Geometry: final body of the model. Coordinates: model frame, mm. Face numbers are marked on the shaded views. A direction names the side the tool comes from. Coordinates: 2 decimals unless noted, no trailing zeros. Loops run counter-clockwise (first coordinate to the right, second up) from the corner with the lowest first, then second, coordinate; pieces in that order, holes last. Notation, with made-up numbers: (57, -27.5) - (104, -27.5) arc R19 ccw to (104, -18.5) - close; hole circle Ø5 at (22.25, -1). An arc over 180 degrees is marked (long way). Answer in a Markdown table with one row per item.
from build123d import *

# Parameters (mm, degrees)
ESBO_O1_R                     = 7.7
ESBO_O1_R_2                   = 5.7
RESSALTO_EXTRUS_O1_DEPTH      = 40
RESSALTO_EXTRUS_O3_DEPTH      = 1
RESSALTO_EXTRUS_O3_DEPTH_BACK = 2
ESBO_O4_R                     = 1.65
CORTE_EXTRUS_O1_DEPTH         = 9.7
ESBO_O5_W                     = 3.890243015
ESBO_O5_H                     = 2
RESSALTO_EXTRUS_O4_DEPTH      = 40
PADR_OCIRCULAR1_COUNT         = 10
ESBO_O6_R                     = 5.3
CORTE_EXTRUS_O2_DEPTH         = 41


with BuildPart() as part:
    # Esboço1 → Ressalto-extrusão1 (new body)
    with BuildSketch(Plane.XY):
        Circle(ESBO_O1_R)
        Circle(ESBO_O1_R_2, mode=Mode.SUBTRACT)
    extrude(amount=RESSALTO_EXTRUS_O1_DEPTH)

    # Esboço3 → Ressalto-extrusão3 (add, two sides)
    with BuildSketch(Plane(origin=(0, 0, 0), x_dir=(1, 0, 0), z_dir=(0, 1, 0))) as ressalto_extrus_o3_sk:
        Polygon((7.7, -40), (13.7, -35), (13.7, -29), (7.7, -24), (6.7, -24), (6.7, -40), align=None)
        Polygon((7.7, 0), (13.7, -5), (13.7, -11), (7.7, -16), (6.7, -16), (6.7, 0), align=None)
        Polygon((-7.7, -28), (-13.7, -23), (-13.7, -17), (-7.7, -12), (-6.7, -12), (-6.7, -28), align=None)
    extrude(amount=RESSALTO_EXTRUS_O3_DEPTH)
    extrude(ressalto_extrus_o3_sk.sketch, amount=-RESSALTO_EXTRUS_O3_DEPTH_BACK)

    # Esboço4 → Corte-extrusão1 (cut, through all)
    with BuildSketch(Plane(origin=(0, 1, 0), x_dir=(1, 0, 0), z_dir=(0, 1, 0))):
        with Locations((10.2, -32)):
            Circle(ESBO_O4_R)
        with Locations((10.2, -8)):
            Circle(ESBO_O4_R)
        with Locations((-10.2, -20)):
            Circle(ESBO_O4_R)
    extrude(amount=-CORTE_EXTRUS_O1_DEPTH, mode=Mode.SUBTRACT)

    # Esboço5 → Ressalto-extrusão4 (add)
    with BuildSketch(Plane.XY.offset(40)):
        with Locations((-4.945121507, 0)):
            Rectangle(ESBO_O5_W, ESBO_O5_H)
    ressalto_extrus_o4 = extrude(amount=-RESSALTO_EXTRUS_O4_DEPTH)

    # PadrãoCircular1: Ressalto-extrusão4 ×10 about axis
    padr_ocircular1_axis = Axis((0, 0, 0), (0, 0, 1))
    for i in range(1, PADR_OCIRCULAR1_COUNT):
        add(ressalto_extrus_o4.rotate(padr_ocircular1_axis, i * 360 / PADR_OCIRCULAR1_COUNT))

    # Esboço6 → Corte-extrusão2 (cut, through all)
    with BuildSketch(Plane.XY.offset(40)):
        Circle(ESBO_O6_R)
    extrude(amount=-CORTE_EXTRUS_O2_DEPTH, mode=Mode.SUBTRACT)


solid = part.part
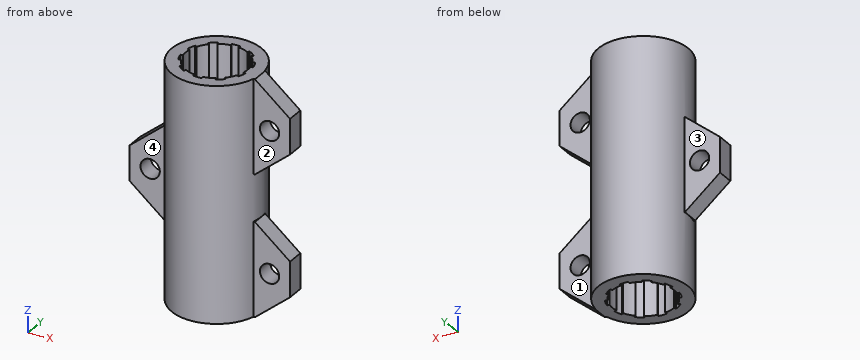
(1) Access query for the marked faces 1, 2, 3 and 4. Directions: +Z, -Z, +X, -X, +Y, -Y. A direction counts if a zero-diameter tool reaches every point of the face in a straight line with its end or side. Return the directions, or none.
Verdict:
| item | result |
|---|---|
| face 1 | +Z, -Z, +X, +Y |
| face 2 | +Z, -Z, +X, -Y |
| face 3 | +Z, -Z, -X, +Y |
| face 4 | +Z, -Z, -X, -Y |
(2) Cut plane B-B on y = -0.5. State how many separate pieces and enclosed holes the cut face has, then the cut area to 3 significant figures.
Verdict:
| item | result |
|---|---|
| separate pieces | 2 |
| enclosed holes | 3 |
| area | 366 mm² |
(3) Cut plane D-D on x = 10.2. Output: boundary loops of the cut face in (y, z), then the cut area to 3 significant figures.
Verdict:
| item | result |
|---|---|
| outline | (-2, 2.08) - (1, 2.08) - (1, 6.35) - (-2, 6.35) - close; (-2, 9.65) - (1, 9.65) - (1, 13.92) - (-2, 13.92) - close; (-2, 26.08) - (1, 26.08) - (1, 30.35) - (-2, 30.35) - close; (-2, 33.65) - (1, 33.65) - (1, 37.92) - (-2, 37.92) - close |
| area | 51.2 mm² |
(4) First-contact query: pin 1 Ø3 at (x, z) = (12, 5.5) entering from -Y; pin 2 Ø6 at (x, y) = (4, 1.5) entering from +Z; pin 3 Ø8 at (x, z) = (5, 34.5) entering from -Y; pin 4 Ø6 at (y, z) = (5.5, 20.5) entering from +X. Flat tips, straight axial feed; report the tip coordinate or a pass-through.
Verdict:
| item | result |
|---|---|
| pin 1 | stops at y = -2 |
| pin 2 | stops at z = 40 |
| pin 3 | stops at y = -7.63 |
| pin 4 | stops at x = 7.28 |
(5) Ray query, probe 1 along X at (y, z) = (0.3, 8); probe 2 along X at (y, z) = (-0.5, 20); probe 3 along X at (y, z) = (-4.75, 30). Return the intervals inside material, ascending.
Verdict:
| item | result |
|---|---|
| probe 1 | x = -7.69 to -5.29, 5.29 to 8.55, 11.85 to 13.7 |
| probe 2 | x = -13.7 to -11.85, -8.55 to -5.28, 5.28 to 7.68 |
| probe 3 | x = -6.06 to -3.15, -2.59 to -2.35, 2.35 to 2.59, 3.15 to 6.06 |
(6) Cut plane A-A on x = 0. Output: boundary loops of the cut face in (y, z), then the cut area to 3 significant figures.
Verdict:
| item | result |
|---|---|
| outline | (-7.7, 0) - (-5.7, 0) - (-5.7, 40) - (-7.7, 40) - close; (5.7, 0) - (7.7, 0) - (7.7, 40) - (5.7, 40) - close |
| area | 160 mm² |
